Input: part model. Units: mm. Frame: model coordinates. A direction names the side the tool comes from. Coordinates: 2 decimals unless noted, no trailing zeros.
1) Pin query (flat end, axial travel): pin 1 Ø5 at (x, y) = (123, -7.5) entering from -Z. Return the tip coordinate at first contact, or that it passes through.
2) Section query A-A (z = 0.7). State how many separate pieces and enclosed holes the cut face has, then the cut area to 3 significant figures.
3) Draft query along X for faces 1 (the cylindrical face through (352.16, -30.15, 1.57)), 2 (the cylindrical face through (245.657, -1.108, 1.565)), 3 (the flat face through (162, 9, 3.175)). Return one class per face: pulls with the +X half, pulls with the -X half, needs draft (parallel to the pull), parting line crosses it, or undercut.
4) Line query: L1, parallel to Y at x = 65, z = 2.55; L2, parallel to Y at x = 320.2, z = 1.4; L3, parallel to X at y = 22, z = 0.95. Output: solid intervals per line, ascending.
5) Set-up query: faces 4 (the flat face through (55.18, 14.68, 1.57)), 5 (the flat face through (372.735, 9.137, 1.565)). Return all of +Z, -Z, +X, -X, +Y, -Y with unobstructed straight access to the full face (end or side cutting, diameter ignored); none if empty.
Autodesk Inventor part; units mm, degrees
ref_plane "YZ Plane" through (0, 0, 0) normal (1, 0, 0) x (0, 1, 0)
ref_plane "XZ Plane" through (0, 0, 0) normal (0, 1, 0) x (-1, 0, 0)
ref_plane "XY Plane" through (0, 0, 0) normal (0, 0, 1) x (1, 0, 0)
sketch "main_sketch" plane through (0, 0, 0) normal (0, 0, 1) x (1, 0, 0)
  circle A0 centre (0, 0) radius 50 construction
  circle A1 centre (330.2, 0) radius 50 construction
  circle A2 centre (0, 0) radius 12.7 construction
  circle A3 centre (330.2, 0) radius 12.7 construction
  circle A4 centre (68.8579, 36.0008) radius 12.7 construction
  circle A5 centre (252.6579, -0.8) radius 12.7 construction
  line L0 (68.8579, 36.0008) -> (0, 0) construction
  circle A6 centre (68.8579, 36.0008) radius 6.75 construction
  circle A7 centre (252.6579, -0.8) radius 6.75 construction
  line L1 (96.8579, 55) -> (220.7349, 55) construction
  line L2 (220.7349, 55) -> (220.7349, 17.0016) construction
  line L3 (220.7349, 17.0016) -> (96.8579, 17.0016) construction
  line L4 (96.8579, 17.0016) -> (96.8579, 55) construction
  line L5 (224.6579, -19.7992) -> (100.7809, -19.7992) construction
  line L6 (100.7809, -19.7992) -> (100.7809, 18.1992) construction
  line L7 (100.7809, 18.1992) -> (224.6579, 18.1992) construction
  line L8 (224.6579, 18.1992) -> (224.6579, -19.7992) construction
  line L9 (100.7809, -0.8) -> (224.6579, -0.8) construction
  line L10 (96.8579, 36.0008) -> (220.7349, 36.0008) construction
  line L11 (330.331, -12.6993) -> (252.7889, -13.4993) construction
  line L12 (5.8842, -11.2546) -> (74.7421, 24.7462) construction
  line L13 (-5.8842, 11.2546) -> (62.9737, 47.2554) construction
  line L14 (254.6579, -13.3) -> (278.6579, -13.3) construction
  line L15 (278.6579, -13.3) -> (278.6579, -37.3) construction
  line L16 (278.6579, -37.3) -> (254.6579, -37.3) construction
  line L17 (254.6579, -37.3) -> (254.6579, -13.3) construction
  line L18 (252.6579, -0.8) -> (330.2, 0) construction
  line L19 (0, -50) -> (330.2, -50) construction
  line L20 (250.6579, -37.3) -> (226.6579, -37.3) construction
  line L21 (226.6579, -37.3) -> (226.6579, -13.3) construction
  line L22 (226.6579, -13.3) -> (250.6579, -13.3) construction
  line L23 (250.6579, -13.3) -> (250.6579, -37.3) construction
  line L24 (-50, 58.175) -> (380.2, 58.175) construction
  line L25 (380.2, 58.175) -> (380.2, 55) construction
  line L26 (380.2, 55) -> (-50, 55) construction
  line L27 (-50, 55) -> (-50, 58.175) construction
  line L28 (252.5269, 11.8993) -> (330.069, 12.6993) construction
  line L29 (224.6579, 8.7) -> (238.5511, 8.7) construction
  line L30 (238.5511, 8.7) -> (238.5511, -10.3) construction
  line L31 (238.5511, -10.3) -> (224.6579, -10.3) construction
  line L32 (224.6579, -10.3) -> (224.6579, 8.7) construction
  line L33 (225.6579, -12.3) -> (279.6579, -12.3)
  line L34 (279.6579, -12.3) -> (279.6579, -37.3)
  line L35 (225.6579, -12.3) -> (225.6579, -37.3)
  line L36 (317.9425, 55) -> (342.8961, 55) construction
  line L37 (342.8961, 55) -> (342.8961, 50) construction
  line L38 (342.8961, 50) -> (317.9425, 50) construction
  line L39 (317.9425, 50) -> (317.9425, 55) construction
  line L40 (380.2, 55) -> (380.2, -5.9093) construction
  line L41 (-50, 55) -> (-50, 17.1992) construction
  line L42 (-50, 55) -> (380.2, 55) construction
  line L43 (-50, 55) -> (380.2, 55)
  circle A8 centre (330.2, 0) radius 14.2748
  circle A9 centre (0, 0) radius 14.2748
  circle A10 centre (252.6579, -0.8) radius 7.008
  circle A11 centre (68.8579, 36.0008) radius 7.008
  circle A12 centre (330.2, 0) radius 37.3
  circle A13 centre (0, 0) radius 37.3
  line L44 (380.2, 52.5) -> (380.2, 43)
  line L45 (380.2, 55) -> (380.2, 31)
  line L46 (380.2, 31) -> (365.4988, -12.0533)
  line L47 (279.6579, -37.3) -> (330.2, -37.3)
  line L48 (-50, 55) -> (-50, 31)
  line L49 (-50, 31) -> (-35.2988, -12.0533)
  line L50 (225.6579, -37.3) -> (0, -37.3)
  circle A14 centre (296.2, 47) radius 2
  circle A15 centre (304.2, 47) radius 2
  circle A16 centre (312.2, 47) radius 2
  circle A17 centre (320.2, 47) radius 2
  circle A18 centre (328.2, 47) radius 2
  circle A19 centre (336.2, 47) radius 2
  circle A20 centre (344.2, 47) radius 2
  circle A21 centre (352.2, 47) radius 2
  circle A22 centre (360.2, 47) radius 2
  circle A23 centre (368.2, 47) radius 2
  circle A24 centre (376.2, 47) radius 2
  circle A25 centre (-46, 47) radius 2
  circle A26 centre (-38, 47) radius 2
  circle A27 centre (-30, 47) radius 2
  circle A28 centre (-22, 47) radius 2
  circle A29 centre (-6, 47) radius 2
  circle A30 centre (-14, 47) radius 2
  circle A31 centre (2, 47) radius 2
  circle A32 centre (10, 47) radius 2
  circle A33 centre (18, 47) radius 2
  circle A34 centre (26, 47) radius 2
  circle A35 centre (34, 47) radius 2
  circle A36 centre (284.6579, -32.3) radius 4
  circle A37 centre (284.6579, -32.3) radius 2
  line L51 (272.5269, 21.8993) -> (272.5269, 1.8993) construction
  line L52 (270.5269, 21.8993) -> (270.5269, 1.8993)
  line L53 (274.5269, 1.8993) -> (274.5269, 21.8993)
  arc A38 (274.5269, 21.8993) -> (270.5269, 21.8993) centre (272.5269, 21.8993) ccw
  arc A39 (270.5269, 1.8993) -> (274.5269, 1.8993) centre (272.5269, 1.8993) ccw
  line L54 (61.6516, 6.6178) -> (52.3851, 24.3416) construction
  line L55 (63.4239, 7.5445) -> (54.1575, 25.2683)
  line L56 (50.6127, 23.415) -> (59.8792, 5.6912)
  arc A40 (59.8792, 5.6912) -> (63.4239, 7.5445) centre (61.6516, 6.6178) ccw
  arc A41 (54.1575, 25.2683) -> (50.6127, 23.415) centre (52.3851, 24.3416) ccw
  circle A42 centre (209.6579, -28.5496) radius 4
  line L57 (221.9902, -19.7992) -> (221.9902, -37.3)
  circle A43 centre (161.6579, -28.5496) radius 4
  circle A44 centre (113.6579, -28.5496) radius 4
  circle A45 centre (65.6579, -28.5496) radius 4
  circle A46 centre (209.6579, -28.5496) radius 2
  circle A47 centre (161.6579, -28.5496) radius 2
  circle A48 centre (113.6579, -28.5496) radius 2
  circle A49 centre (65.6579, -28.5496) radius 2
  circle A50 centre (252.6579, 36.0008) radius 4
  circle A51 centre (252.6579, 36.0008) radius 2
  point P0 (238.5511, -0.8)
  point P1 (272.5269, 11.8993)
  point P2 (57.0183, 15.4797)
  point P3 (221.9902, -28.5496)
  dimension "d0" = 100
  dimension "d1" = 100
  dimension "d2" = 25.4
  dimension "d3" = 25.4
  dimension "d4" = 25.4
  dimension "d5" = 25.4
  dimension "d6" = 13.5
  dimension "d7" = 13.5
  dimension "d8" = 37.9984
  dimension "d9" = 37.9984
  dimension "d10" = 24
  dimension "d11" = 24
  dimension "d12" = 77.5462
  dimension "d13" = 330.2
  dimension "d14" = 123.877
  dimension "d15" = 123.877
  dimension "d16" = 28
  dimension "d17" = 28
  dimension "d18" = 77.7011
  dimension "d19" = 12.7
  dimension "d20" = 24
  dimension "d21" = 3.175
  dimension "d23" = 12.7
  dimension "d24" = 4
  dimension "d25" = 19
  dimension "d26" = 1
  dimension "d27" = 1
  dimension "d28" = 1
  dimension "d29" = 1
  dimension "d32" = 5
  dimension "d34" = 2
  dimension "d40" = 28.5496
  dimension "d41" = 28.5496
  dimension "d42" = 14.016
  dimension "d43" = 14.016
  dimension "d45" = 24
  dimension "d46" = 24
  dimension "d48" = 8
  dimension "d49" = 5
  dimension "d50" = 5
  dimension "d51" = 4
  dimension "d52" = 4
  dimension "d53" = 20
  dimension "d54" = 20
  dimension "d55" = 4
  dimension "d56" = 20
  dimension "d57" = 18
  dimension "d58" = 8
  dimension "d59" = 16
  dimension "d62" = 48
  dimension "d67" = 4
  dimension "d68" = 4
  dimension "d69" = 4
  dimension "d70" = 4
  dimension "d71" = 8
  dimension "d72" = 4
extrude "Extrusion1" add sketch "main_sketch" along normal blind 3.175 contours L35 L50 A13 L49 L48 L43 L45 L44 L46 A12 L47 L34 L33 | A12 | A13 | A36 | A42 | A43 | A44 | A45 | A50
fillet "Fillet4" radius 4 4 edges at (279.6579, -37.3, 1.5875) (279.6579, -12.3, 1.5875) (225.6579, -12.3, 1.5875) (225.6579, -37.3, 1.5875)
fillet "Fillet5" radius 8 2 edges at (-50, 31, 1.5875) (380.2, 31, 1.5875)
sketch "Sketch3" plane through (0, 0, 3.175) normal (0, 0, 1) x (1, 0, 0)
  line L0 (40.2299, 50.35) -> (218.0299, 50.35) construction
  line L1 (218.0299, 50.35) -> (218.0299, -25.85) construction
  line L2 (218.0299, -25.85) -> (40.2299, -25.85) construction
  line L3 (40.2299, -25.85) -> (40.2299, 50.35) construction
  circle A0 centre (40.2299, 50.35) radius 1.65
  circle A1 centre (218.0299, 50.35) radius 1.65
  circle A2 centre (40.2299, -25.85) radius 1.65
  circle A3 centre (218.0299, -25.85) radius 1.65
  line L4 (380.2, 55) -> (-50, 55)
  circle A4 centre (68.8579, 36.0008) radius 7.008
  point P0 (0, 0)
  dimension "d109" = 177.8
  dimension "d110" = 76.2
  dimension "d111" = 3.3
  dimension "d112" = 3.3
  dimension "d113" = 3.3
  dimension "d114" = 3.3
  dimension "d115" = 4.65
extrude "Extrusion2" cut sketch "Sketch3" against normal through all contours A0 | A1 | A2 | A3
equation "\"d9\" = d8"
equation "\"d15\" = d14"
equation "\"d20\" = d10"
properties part number "outside_plate"
Answer:
1. pin 1: stops at z = 0
2. separate pieces: 1
2. enclosed holes: 38
2. area: 34,300 mm2
3. face 1: pulls with the +X half
3. face 2: undercut
3. face 3: needs draft
4. L1: y = -37.3 to -30.44, -26.66 to 30.15, 41.85 to 55
4. L2: y = -37.3 to -10.19, 10.19 to 45, 49 to 55
4. L3: x = -46.93 to 51.35, 55.87 to 270.53, 274.52 to 377.13
5. face 4: +Z, -Z
5. face 5: +Z, -Z, +X, -Y
